Design review of the part built by this model. Coordinates are the model's own, in mm. Face numbers are marked on the shaded views. A direction names the side the tool comes from. Coordinates: 2 decimals unless noted, no trailing zeros. Write each loop counter-clockwise with the first axis right and the second up, starting at its lowest first coordinate (ties: lowest second). Pieces come first, ordered by that corner, then holes. Notation, with made-up numbers: (-11.5, 47) - (-2.5, 47) arc R19 cw to (-2.5, 57) - close; hole circle Ø2 at (-22, 15). An arc over 180 degrees is marked (long way). Answer as a JSON object with one key per item and string values.
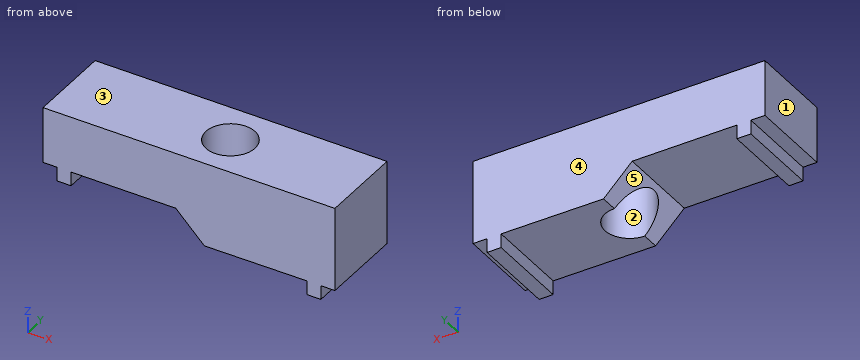
```python
from build123d import *

# Parameters (mm, degrees)
F1_DEPTH      = 6
F2_R          = 1.75
F3_DEPTH      = 4.001
F3_DEPTH_BACK = 3.001


# Not quite as in the source:
# - a feature of the source that left no trace in its solid (it failed there, or was rolled back) is left out


with BuildPart() as f1:
    # F0 (on Front) → F1 (new body)
    with BuildSketch(Plane.XZ):
        Polygon((20.8, 0), (0, 0), (0, -4), (1, -4), (1, -5), (2, -5), (2, -4), (9.4564415496, -4), (11.5, -6.0279625468), (18.8, -6), (18.8, -7), (19.8, -7), (19.8, -6), (20.8, -6), align=None)
    extrude(amount=F1_DEPTH)

    # F2 (on face) → F3 (cut, two sides)
    with BuildSketch(Plane(origin=(0, 0, -4), x_dir=(1, 0, 0), z_dir=(0, 0, -1))) as f3_sk:
        with Locations((11.5, 3)):
            Circle(F2_R)
    extrude(amount=-F3_DEPTH, mode=Mode.SUBTRACT)
    extrude(f3_sk.sketch, amount=F3_DEPTH_BACK, mode=Mode.SUBTRACT)


solid = f1.part
```
(1) Take a section at D-D, the plane y = -0.6. Write out the cut boundary in (x, z), and give its area (3 significant figures).
Solved:
{"outline": "(0, -4) - (1, -4) - (1, -5) - (2, -5) - (2, -4) - (9.46, -4) - (11.5, -6.03) - (18.8, -6) - (18.8, -7) - (19.8, -7) - (19.8, -6) - (20.8, -6) - (20.8, 0) - (0, 0) - close", "area": "106 mm^2"}
(2) Take a section at A-A, the plane y = -2.45. Write out the cut boundary in (x, z).
Solved:
{"outline": "(0, -4) - (1, -4) - (1, -5) - (2, -5) - (2, -4) - (9.46, -4) - (9.84, -4.38) - (9.84, 0) - (0, 0) - close; (13.16, -6.02) - (18.8, -6) - (18.8, -7) - (19.8, -7) - (19.8, -6) - (20.8, -6) - (20.8, 0) - (13.16, 0) - close"}
(3) Take a section at C-C, the plane x = 12.5. Write out the cut boundary in (y, z), and give its area (3 significant figures).
Solved:
{"outline": "(-6, -6.02) - (-4.44, -6.02) - (-4.44, 0) - (-6, 0) - close; (-1.56, -6.02) - (0, -6.02) - (0, 0) - (-1.56, 0) - close", "area": "18.8 mm^2"}
(4) For pin 1 (1.1 mm diameter, centred on x = 0.5, y = -2, fed in from -Z); pin 2 (1.8 mm diameter, centred on x = 5.5, y = -1.5, fed in from -Z); pin 3 (1.1 mm diameter, centred on x = 20.5, y = -3.5, fed in from -Z), all flat-tipped, find the tip position at first contact; note any pin that passes through.
Solved:
{"pin 1": "stops at z = -5", "pin 2": "stops at z = -4", "pin 3": "stops at z = -6"}
(5) To check wall thickness, follow line 1 (X direction, y = -3, z = -4.5); line 2 (X direction, y = -3, z = -2); line 3 (Y direction, x = 11.5, z = -4). State the ranges of each line that lie inside material, in increasing order. Write a range as from..to.
Solved:
{"line 1": "x = 1..2, 13.25..20.8", "line 2": "x = 0..9.75, 13.25..20.8", "line 3": "y = -6..-4.75, -1.25..0"}
(6) Take a section at B-B, the plane z = -1. Write out the cut boundary in (x, y).
Solved:
{"outline": "(0, -6) - (20.8, -6) - (20.8, 0) - (0, 0) - close; hole circle Ø3.5 at (11.5, -3)"}
(7) Tool access review of the marked faces 4 and 5: name each direction out of +Z, -Z, +X, -X, +Y, -Y from which nothing blocks a thin tool from reaching the whole face with its end or side.
Solved:
{"face 4": "+Z, -Z, +X, -X, +Y", "face 5": "-Z, +Y, -Y"}
(8) The part is to be moulded in two halves that separate along X. For the marked faces 1, 2 and 3, say which applies: pulls with the +X half, pulls with the -X half, needs draft (parallel to the pull), parting line crosses it, or undercut.
Solved:
{"face 1": "pulls with the -X half", "face 2": "undercut", "face 3": "needs draft"}
